from build123d import *

# Parameters (mm, degrees)
CROQUIS1_W              = 28
CROQUIS1_H              = 8
CROQUIS1_R              = 2.85
CROQUIS1_R_2            = 1.5
SALIENTE_EXTRUIR1_DEPTH = 4
CORTAR_EXTRUIR1_START   = 2.35
CROQUIS1_3_R            = 2.85
CORTAR_EXTRUIR1_DEPTH   = 13.749668871
CROQUIS2_W              = 12
CROQUIS2_H              = 4
SALIENTE_EXTRUIR2_DEPTH = 40
CROQUIS3_W              = 12
CROQUIS3_H              = 8
SALIENTE_EXTRUIR3_DEPTH = 10
CROQUIS4_W              = 4.4
CROQUIS4_H              = 8
CORTAR_EXTRUIR2_DEPTH   = 57.356011214
CORTAR_EXTRUIR7_START   = -12
CROQUIS5_R              = 1.5
CORTAR_EXTRUIR7_DEPTH   = 12
CORTAR_EXTRUIR8_START   = -1.54
CROQUIS5_4_R            = 2.85
CROQUIS5_4_R_2          = 1.5
CORTAR_EXTRUIR8_DEPTH   = 1.54
CORTAR_EXTRUIR9_DEPTH   = 2
SALIENTE_EXTRUIR4_DEPTH = 12


with BuildPart() as part:
    # Croquis1 → Saliente-Extruir1 (new body)
    # profile 1 of 3: a face of its own
    with BuildSketch(Plane(origin=(0, 0, 0), x_dir=(1, 0, 0), z_dir=(0, 1, 0))):
        Rectangle(CROQUIS1_W, CROQUIS1_H)
        with Locations((-10, 0)):
            Circle(CROQUIS1_R, mode=Mode.SUBTRACT)
        with Locations((10, 0)):
            Circle(CROQUIS1_R, mode=Mode.SUBTRACT)
    # profile 2 of 3: a face of its own
    with BuildSketch(Plane(origin=(0, 0, 0), x_dir=(1, 0, 0), z_dir=(0, 1, 0))):
        with Locations((-10, 0)):
            Circle(CROQUIS1_R)
        with Locations(Location((-10, 0, 0), (0, 0, 270))):
            Circle(CROQUIS1_R_2, mode=Mode.SUBTRACT)
    # profile 3 of 3: a face of its own
    with BuildSketch(Plane(origin=(0, 0, 0), x_dir=(1, 0, 0), z_dir=(0, 1, 0))):
        with Locations((10, 0)):
            Circle(CROQUIS1_R)
        with Locations(Location((10, 0, 0), (0, 0, 270))):
            Circle(CROQUIS1_R_2, mode=Mode.SUBTRACT)
    extrude(amount=SALIENTE_EXTRUIR1_DEPTH)

    # Croquis1<3> → Cortar-Extruir1 (cut, through all)
    with BuildSketch(Plane(origin=(0, 0, 0), x_dir=(1, 0, 0), z_dir=(0, 1, 0)).offset(CORTAR_EXTRUIR1_START)):
        with Locations(Location((-10, 0, 0), (0, 0, 270))):
            Circle(CROQUIS1_3_R)
        with Locations(Location((10, 0, 0), (0, 0, 90))):
            Circle(CROQUIS1_3_R)
    extrude(amount=CORTAR_EXTRUIR1_DEPTH, mode=Mode.SUBTRACT)

    # Croquis2 → Saliente-Extruir2 (add)
    with BuildSketch(Plane(origin=(0, 4, 0), x_dir=(1, 0, 0), z_dir=(0, 1, 0))):
        Rectangle(CROQUIS2_W, CROQUIS2_H)
    extrude(amount=SALIENTE_EXTRUIR2_DEPTH)

    # Croquis3 → Saliente-Extruir3 (add)
    with BuildSketch(Plane(origin=(0, 44, 0), x_dir=(1, 0, 0), z_dir=(0, 1, 0))):
        Rectangle(CROQUIS3_W, CROQUIS3_H)
    extrude(amount=SALIENTE_EXTRUIR3_DEPTH)

    # Croquis4 → Cortar-Extruir2 (cut, through all)
    with BuildSketch(Plane.XY.offset(4)):
        with Locations((0, 50)):
            Rectangle(CROQUIS4_W, CROQUIS4_H)
    extrude(amount=-CORTAR_EXTRUIR2_DEPTH, mode=Mode.SUBTRACT)

    # Croquis5 → Cortar-Extruir7 (cut)
    with BuildSketch(Plane.ZY.offset(6).offset(CORTAR_EXTRUIR7_START)):
        with Locations((0, 50)):
            Circle(CROQUIS5_R)
    extrude(amount=CORTAR_EXTRUIR7_DEPTH, mode=Mode.SUBTRACT)

    # Croquis5<4> → Cortar-Extruir8 (cut)
    with BuildSketch(Plane.ZY.offset(6).offset(CORTAR_EXTRUIR8_START)):
        with Locations((0, 50)):
            Circle(CROQUIS5_4_R)
        with Locations((0, 50)):
            Circle(CROQUIS5_4_R_2, mode=Mode.SUBTRACT)
    extrude(amount=CORTAR_EXTRUIR8_DEPTH, mode=Mode.SUBTRACT)

    # Croquis7 → Cortar-Extruir9 (cut)
    with BuildSketch(Plane(origin=(6, 0, 0), x_dir=(0, 0, -1), z_dir=(1, 0, 0))):
        Polygon((-3.406366588, 50), (-1.703183294, 47.05), (1.703183294, 47.05), (3.406366588, 50), (1.703183294, 52.95), (-1.703183294, 52.95), align=None)
    extrude(amount=-CORTAR_EXTRUIR9_DEPTH, mode=Mode.SUBTRACT)

    # Croquis8 → Saliente-Extruir4 (add)
    with BuildSketch(Plane(origin=(6, 0, 0), x_dir=(0, 0, -1), z_dir=(1, 0, 0))):
        Polygon((-4, 44), (-2, 44), (-2, 42.5), align=None)
        Polygon((2, 42.5), (4, 44), (2, 44), align=None)
    extrude(amount=-SALIENTE_EXTRUIR4_DEPTH)


solid = part.part
Model file for the job. Use its own axes, mm. A direction names the side the tool comes from. Coordinates: 2 decimals unless noted, no trailing zeros. Loops run counter-clockwise (first coordinate to the right, second up) from the corner with the lowest first, then second, coordinate; pieces in that order, holes last. Notation, with made-up numbers: (69.5, 49.5) -> (94.5, 49.5) arc R25 cw to (94.5, 81.5) -> close; hole circle Ø1 at (62.5, -30). An arc over 180 degrees is marked (long way). Use one line per item in the form item = value. Start each with the question number.
(1) Probe probe 1 along X at (y, z) = (3.65, 0); probe 2 along X at (y, z) = (50, 1.75); probe 3 along X at (y, z) = (1.75, 0). List the from-to ranges inside material, lowest first. Write a range as from..to.
(2) Cut at D-D on x = -1.25. Give the cut face in (y, z), and give its area (3 significant figures).
(3) Flat gauge pins, fed straight in: pin 1 (4 mm diameter, centred on y = 50, z = 0, fed in from -X); pin 2 (2.5 mm diameter, centred on x = -10, z = 0, fed in from -Y); pin 3 (1 mm diameter, centred on y = 43, z = 0, fed in from -X); pin 4 (2.5 mm diameter, centred on y = 49.5, z = 1.5, fed in from +X). Where does each tip first touch, or does it go through?
(4) Cut at A-A on x = -10. Give the cut face in (y, z).
(5) Pull direction Z, two halves, no side cores. Call faces 5 (the flat face through (14, 2, 0)), 6 (the flat face through (3, 49, -4)), 7 (the flat face through (5.01, 48.55, 2.57)): pulls with the +Z half, pulls with the -Z half, needs draft (parallel to the pull), parting line crosses it, or undercut.
(6) Tool access for faces 1 (the cylindrical face through (-7.174, 3.163, -0.371)), 2 (the flat face through (0, 23, -2)), 3 (the flat face through (0, 23, 2)), 4 (the flat face through (5, 47.05, 0)): list every direction of +Z, -Z, +X, -X, +Y, -Y with a clear straight run to the whole face (end or side of a thin tool).
(7) Cut at B-B on y = 49.5. Give the cut face in (x, z), and give its area (3 significant figures).
(8) Cut at C-C on z = 0. Give the number of separate pieces and of enclosed holes in the cut face, and give its area (3 significant figures).
Values:
q1.probe_1 = -14..-12.85, -7.15..7.15, 12.85..14
q1.probe_2 = -4.46..-2.2, 2.2..4
q1.probe_3 = -14..-11.5, -8.5..8.5, 11.5..14
q2.outline = (0, -4) -> (4, -4) -> (4, -2) -> (42.5, -2) -> (44, -4) -> (46, -4) -> (46, 4) -> (44, 4) -> (42.5, 2) -> (4, 2) -> (4, 4) -> (0, 4) -> close
q2.area = 211 mm2
q3.pin_1 = -4.46
q3.pin_2 = through
q3.pin_3 = -6
q3.pin_4 = 4
q4.outline = (0, -4) -> (4, -4) -> (4, -2.85) -> (2.35, -2.85) -> (2.35, -1.5) -> (0, -1.5) -> close; (0, 1.5) -> (2.35, 1.5) -> (2.35, 2.85) -> (4, 2.85) -> (4, 4) -> (0, 4) -> close
q5.face_5 = needs draft
q5.face_6 = pulls with the -Z half
q5.face_7 = undercut
q6.face_1 = +Y
q6.face_2 = -Z, +X, -X
q6.face_3 = +Z, +X, -X
q6.face_4 = +X
q7.outline = (-6, -4) -> (-2.2, -4) -> (-2.2, -1.41) -> (-4.46, -1.41) -> (-4.46, -2.81) -> (-6, -2.81) -> close; (-6, 2.81) -> (-4.46, 2.81) -> (-4.46, 1.41) -> (-2.2, 1.41) -> (-2.2, 4) -> (-6, 4) -> close; (2.2, -4) -> (6, -4) -> (6, -3.12) -> (4, -3.12) -> (4, -1.41) -> (2.2, -1.41) -> close; (2.2, 1.41) -> (4, 1.41) -> (4, 3.12) -> (6, 3.12) -> (6, 4) -> (2.2, 4) -> close
q7.area = 28.2 mm2
q8.separate_pieces = 5
q8.enclosed_holes = 0
q8.area = 611 mm2
